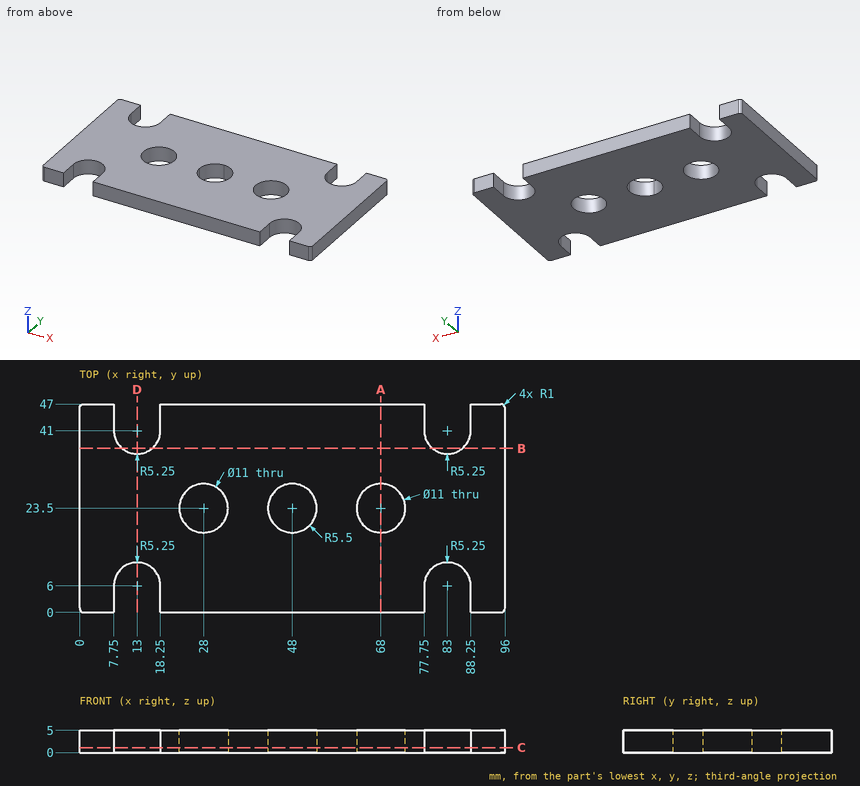
The figure shows three views and two pictorial views of one solid part (mm, origin at its lowest corner). Answer the questions. Coordinates: 2 decimals unless noted, no trailing zeros. Loops run counter-clockwise (first coordinate to the right, second up) from the corner with the lowest first, then second, coordinate; pieces in that order, holes last. Notation, with made-up numbers: (-22, -38) - (14, -38) arc R21 ccw to (14, -14) - close; hole circle Ø10 at (26.25, 81.5). An arc over 180 degrees is marked (long way). Use a Markdown table: item, result. Add a question column.
1) The part is cut by section A-A, the plane x = 68. Give the vertices of the cut face in (y, z).
2) Find the intervals of material crossed by line 1 (X direction, y = 45.5, z = 2.65); line 2 (X direction, y = 25, z = 0.6); line 3 (Y direction, x = 28, z = 1.1), in increasing order.
3) Given pin 1 (6 mm diameter, centred on x = 69.5, y = 7, fed in from -Z), flat-ended and moving along its own axis, determine where the tip first touches the part or whether it passes through.
4) The part is cut by section C-C, the plane z = 1.1. Give the vertices of the cut face in (x, y), and give its area (3 significant figures).
5) The part is cut by section D-D, the plane x = 13. Give the vertices of the cut face in (y, z).
6) The part is cut by section B-B, the plane y = 37. Give the vertices of the cut face in (x, z).
Here are the results:
| question | item | result |
|---|---|---|
| 1 | outline | (0, 0) - (18, 0) - (18, 5) - (0, 5) - close; (29, 0) - (47, 0) - (47, 5) - (29, 5) - close |
| 2 | line 1 | x = 0 to 7.75, 18.25 to 77.75, 88.25 to 96 |
| 2 | line 2 | x = 0 to 22.71, 33.29 to 42.71, 53.29 to 62.71, 73.29 to 96 |
| 2 | line 3 | y = 0 to 18, 29 to 47 |
| 3 | pin 1 | stops at z = 0 |
| 4 | outline | (0, 1) arc R1 ccw to (1, 0) - (7.75, 0) - (7.75, 6) arc R5.25 cw to (18.25, 6) - (18.25, 0) - (77.75, 0) - (77.75, 6) arc R5.25 cw to (88.25, 6) - (88.25, 0) - (95, 0) arc R1 ccw to (96, 1) - (96, 46) arc R1 ccw to (95, 47) - (88.25, 47) - (88.25, 41) arc R5.25 cw to (77.75, 41) - (77.75, 47) - (18.25, 47) - (18.25, 41) arc R5.25 cw to (7.75, 41) - (7.75, 47) - (1, 47) arc R1 ccw to (0, 46) - close; hole circle Ø11 at (28, 23.5); hole circle Ø11 at (48, 23.5); hole circle Ø11 at (68, 23.5) |
| 4 | area | 3,800 mm^2 |
| 5 | outline | (11.25, 0) - (35.75, 0) - (35.75, 5) - (11.25, 5) - close |
| 6 | outline | (0, 0) - (9.6, 0) - (9.6, 5) - (0, 5) - close; (16.4, 0) - (79.6, 0) - (79.6, 5) - (16.4, 5) - close; (86.4, 0) - (96, 0) - (96, 5) - (86.4, 5) - close |
